For this review, take the finished solid that the model builds, in its own axes (mm). A direction names the side the tool comes from. Give positions to 0.01 mm unless a question says otherwise; leave off trailing zeros. Answer in a Markdown table with one row per item.
```python
from build123d import *

# Parameters (mm, degrees)
SKETCH_1_R          = 23.515666667
SKETCH_1_R_2        = 15.01
EXTRUDE_1_DEPTH     = 3
SKETCH_2_R          = 23.515666667
SKETCH_2_R_2        = 22.515666667
CUT_EXTRUDE_3_DEPTH = 1
FILLET_1_R          = 1
FILLET_2_R          = 1
FILLET_3_R          = 1
CUT_EXTRUDE_4_DEPTH = 34.391213778
SKETCH_5_R          = 21.515666667
SKETCH_5_R_2        = 20.515666667
EXTRUDE_2_DEPTH     = 5
EXTRUDE_3_DEPTH     = 2


with BuildPart() as part:
    # 草图1 → 凸台-拉伸1 (new body)
    with BuildSketch(Plane.XY):
        Circle(SKETCH_1_R)
        Circle(SKETCH_1_R_2, mode=Mode.SUBTRACT)
    extrude(amount=EXTRUDE_1_DEPTH)

    # 草图2 → 切除-拉伸3 (cut)
    with BuildSketch(Plane(origin=(0, 0, 0), x_dir=(-1, 0, 0), z_dir=(0, 0, -1))):
        Circle(SKETCH_2_R)
        Circle(SKETCH_2_R_2, mode=Mode.SUBTRACT)
    extrude(amount=-CUT_EXTRUDE_3_DEPTH, mode=Mode.SUBTRACT)

    # 圆角1
    fillet_1_edges = [part.edges().sort_by_distance(p)[0] for p in [
        (-23.515666667, 0, 3),
    ]]
    fillet(fillet_1_edges, radius=FILLET_1_R)

    # 圆角2
    fillet_2_edges = [part.edges().sort_by_distance(p)[0] for p in [
        (-15.01, 0, 3),
    ]]
    fillet(fillet_2_edges, radius=FILLET_2_R)

    # 圆角3
    fillet_3_edges = [part.edges().sort_by_distance(p)[0] for p in [
        (-15.01, 0, 0),
    ]]
    fillet(fillet_3_edges, radius=FILLET_3_R)

    # 草图3 → 切除-拉伸4 (cut, through all)
    with BuildSketch(Plane.XY.offset(3)):
        with BuildLine():
            Line((1.1, 19.35), (1.1, 17.85))
            ThreePointArc((1.1, 17.85), (0, 16.75), (-1.1, 17.85))
            Line((-1.1, 17.85), (-1.1, 19.35))
            ThreePointArc((-1.1, 19.35), (0, 20.45), (1.1, 19.35))
        make_face()
        with BuildLine():
            Line((7.025641009, 18.063024896), (6.562115518, 16.636440122))
            ThreePointArc((6.562115518, 16.636440122), (5.176034656, 15.930196648), (4.469791182, 17.31627751))
            Line((4.469791182, 17.31627751), (4.933316673, 18.742862284))
            ThreePointArc((4.933316673, 18.742862284), (6.319397535, 19.449105758), (7.025641009, 18.063024896))
        make_face()
        with BuildLine():
            Line((12.263563326, 15.007915064), (11.381885447, 13.794389572))
            ThreePointArc((11.381885447, 13.794389572), (9.845402976, 13.551034656), (9.60204806, 15.087517127))
            Line((9.60204806, 15.087517127), (10.483725938, 16.301042619))
            ThreePointArc((10.483725938, 16.301042619), (12.020208409, 16.544397535), (12.263563326, 15.007915064))
        make_face()
        with BuildLine():
            Line((16.301042619, 10.483725938), (15.087517127, 9.60204806))
            ThreePointArc((15.087517127, 9.60204806), (13.551034656, 9.845402976), (13.794389572, 11.381885447))
            Line((13.794389572, 11.381885447), (15.007915064, 12.263563326))
            ThreePointArc((15.007915064, 12.263563326), (16.544397535, 12.020208409), (16.301042619, 10.483725938))
        make_face()
        with BuildLine():
            Line((18.742862284, 4.933316673), (17.31627751, 4.469791182))
            ThreePointArc((17.31627751, 4.469791182), (15.930196648, 5.176034656), (16.636440122, 6.562115518))
            Line((16.636440122, 6.562115518), (18.063024896, 7.025641009))
            ThreePointArc((18.063024896, 7.025641009), (19.449105758, 6.319397535), (18.742862284, 4.933316673))
        make_face()
        with BuildLine():
            Line((19.35, -1.1), (17.85, -1.1))
            ThreePointArc((17.85, -1.1), (16.75, 0), (17.85, 1.1))
            Line((17.85, 1.1), (19.35, 1.1))
            ThreePointArc((19.35, 1.1), (20.45, 0), (19.35, -1.1))
        make_face()
        with BuildLine():
            Line((18.063024896, -7.025641009), (16.636440122, -6.562115518))
            ThreePointArc((16.636440122, -6.562115518), (15.930196648, -5.176034656), (17.31627751, -4.469791182))
            Line((17.31627751, -4.469791182), (18.742862284, -4.933316673))
            ThreePointArc((18.742862284, -4.933316673), (19.449105758, -6.319397535), (18.063024896, -7.025641009))
        make_face()
        with BuildLine():
            Line((15.007915064, -12.263563326), (13.794389572, -11.381885447))
            ThreePointArc((13.794389572, -11.381885447), (13.551034656, -9.845402976), (15.087517127, -9.60204806))
            Line((15.087517127, -9.60204806), (16.301042619, -10.483725938))
            ThreePointArc((16.301042619, -10.483725938), (16.544397535, -12.020208409), (15.007915064, -12.263563326))
        make_face()
        with BuildLine():
            Line((10.483725938, -16.301042619), (9.60204806, -15.087517127))
            ThreePointArc((9.60204806, -15.087517127), (9.845402976, -13.551034656), (11.381885447, -13.794389572))
            Line((11.381885447, -13.794389572), (12.263563326, -15.007915064))
            ThreePointArc((12.263563326, -15.007915064), (12.020208409, -16.544397535), (10.483725938, -16.301042619))
        make_face()
        with BuildLine():
            Line((4.933316673, -18.742862284), (4.469791182, -17.31627751))
            ThreePointArc((4.469791182, -17.31627751), (5.176034656, -15.930196648), (6.562115518, -16.636440122))
            Line((6.562115518, -16.636440122), (7.025641009, -18.063024896))
            ThreePointArc((7.025641009, -18.063024896), (6.319397535, -19.449105758), (4.933316673, -18.742862284))
        make_face()
        with BuildLine():
            Line((-1.1, -19.35), (-1.1, -17.85))
            ThreePointArc((-1.1, -17.85), (0, -16.75), (1.1, -17.85))
            Line((1.1, -17.85), (1.1, -19.35))
            ThreePointArc((1.1, -19.35), (0, -20.45), (-1.1, -19.35))
        make_face()
        with BuildLine():
            Line((-7.025641009, -18.063024896), (-6.562115518, -16.636440122))
            ThreePointArc((-6.562115518, -16.636440122), (-5.176034656, -15.930196648), (-4.469791182, -17.31627751))
            Line((-4.469791182, -17.31627751), (-4.933316673, -18.742862284))
            ThreePointArc((-4.933316673, -18.742862284), (-6.319397535, -19.449105758), (-7.025641009, -18.063024896))
        make_face()
        with BuildLine():
            Line((-12.263563326, -15.007915064), (-11.381885447, -13.794389572))
            ThreePointArc((-11.381885447, -13.794389572), (-9.845402976, -13.551034656), (-9.60204806, -15.087517127))
            Line((-9.60204806, -15.087517127), (-10.483725938, -16.301042619))
            ThreePointArc((-10.483725938, -16.301042619), (-12.020208409, -16.544397535), (-12.263563326, -15.007915064))
        make_face()
        with BuildLine():
            Line((-16.301042619, -10.483725938), (-15.087517127, -9.60204806))
            ThreePointArc((-15.087517127, -9.60204806), (-13.551034656, -9.845402976), (-13.794389572, -11.381885447))
            Line((-13.794389572, -11.381885447), (-15.007915064, -12.263563326))
            ThreePointArc((-15.007915064, -12.263563326), (-16.544397535, -12.020208409), (-16.301042619, -10.483725938))
        make_face()
        with BuildLine():
            Line((-18.742862284, -4.933316673), (-17.31627751, -4.469791182))
            ThreePointArc((-17.31627751, -4.469791182), (-15.930196648, -5.176034656), (-16.636440122, -6.562115518))
            Line((-16.636440122, -6.562115518), (-18.063024896, -7.025641009))
            ThreePointArc((-18.063024896, -7.025641009), (-19.449105758, -6.319397535), (-18.742862284, -4.933316673))
        make_face()
        with BuildLine():
            Line((-19.35, 1.1), (-17.85, 1.1))
            ThreePointArc((-17.85, 1.1), (-16.75, 0), (-17.85, -1.1))
            Line((-17.85, -1.1), (-19.35, -1.1))
            ThreePointArc((-19.35, -1.1), (-20.45, 0), (-19.35, 1.1))
        make_face()
        with BuildLine():
            Line((-18.063024896, 7.025641009), (-16.636440122, 6.562115518))
            ThreePointArc((-16.636440122, 6.562115518), (-15.930196648, 5.176034656), (-17.31627751, 4.469791182))
            Line((-17.31627751, 4.469791182), (-18.742862284, 4.933316673))
            ThreePointArc((-18.742862284, 4.933316673), (-19.449105758, 6.319397535), (-18.063024896, 7.025641009))
        make_face()
        with BuildLine():
            Line((-15.007915064, 12.263563326), (-13.794389572, 11.381885447))
            ThreePointArc((-13.794389572, 11.381885447), (-13.551034656, 9.845402976), (-15.087517127, 9.60204806))
            Line((-15.087517127, 9.60204806), (-16.301042619, 10.483725938))
            ThreePointArc((-16.301042619, 10.483725938), (-16.544397535, 12.020208409), (-15.007915064, 12.263563326))
        make_face()
        with BuildLine():
            Line((-10.483725938, 16.301042619), (-9.60204806, 15.087517127))
            ThreePointArc((-9.60204806, 15.087517127), (-9.845402976, 13.551034656), (-11.381885447, 13.794389572))
            Line((-11.381885447, 13.794389572), (-12.263563326, 15.007915064))
            ThreePointArc((-12.263563326, 15.007915064), (-12.020208409, 16.544397535), (-10.483725938, 16.301042619))
        make_face()
        with BuildLine():
            Line((-4.933316673, 18.742862284), (-4.469791182, 17.31627751))
            ThreePointArc((-4.469791182, 17.31627751), (-5.176034656, 15.930196648), (-6.562115518, 16.636440122))
            Line((-6.562115518, 16.636440122), (-7.025641009, 18.063024896))
            ThreePointArc((-7.025641009, 18.063024896), (-6.319397535, 19.449105758), (-4.933316673, 18.742862284))
        make_face()
    extrude(amount=-CUT_EXTRUDE_4_DEPTH, mode=Mode.SUBTRACT)

    # 草图5 → 凸台-拉伸2 (add)
    with BuildSketch(Plane(origin=(0, 0, 0), x_dir=(-1, 0, 0), z_dir=(0, 0, -1))):
        with Locations(Location((0, 0, 0), (0, 0, 180))):
            Circle(SKETCH_5_R)
        Circle(SKETCH_5_R_2, mode=Mode.SUBTRACT)
    extrude(amount=EXTRUDE_2_DEPTH)

    # 草图6 → 凸台-拉伸3 (add)
    with BuildSketch(Plane(origin=(0, 0, -5), x_dir=(-1, 0, 0), z_dir=(0, 0, -1))):
        with BuildLine():
            Line((-16.26911987, -9.852722397), (-18.353991972, -11.115339319))
            ThreePointArc((-18.353991972, -11.115339319), (-20.274508623, -7.025958268), (-21.29621173, -2.625101039))
            Line((-21.29621173, -2.625101039), (-18.877126128, -2.326909783))
            ThreePointArc((-18.877126128, -2.326909783), (-17.971480624, -6.227863532), (-16.26911987, -9.852722397))
        make_face()
        with BuildLine():
            Line((-9.852722397, 16.26911987), (-11.115339319, 18.353991972))
            ThreePointArc((-11.115339319, 18.353991972), (-7.025958268, 20.274508623), (-2.625101039, 21.29621173))
            Line((-2.625101039, 21.29621173), (-2.326909783, 18.877126128))
            ThreePointArc((-2.326909783, 18.877126128), (-6.227863532, 17.971480624), (-9.852722397, 16.26911987))
        make_face()
        with BuildLine():
            Line((16.26911987, 9.852722397), (18.353991972, 11.115339319))
            ThreePointArc((18.353991972, 11.115339319), (20.274508623, 7.025958268), (21.29621173, 2.625101039))
            Line((21.29621173, 2.625101039), (18.877126128, 2.326909783))
            ThreePointArc((18.877126128, 2.326909783), (17.971480624, 6.227863532), (16.26911987, 9.852722397))
        make_face()
        with BuildLine():
            Line((9.852722397, -16.26911987), (11.115339319, -18.353991972))
            ThreePointArc((11.115339319, -18.353991972), (7.025958268, -20.274508623), (2.625101039, -21.29621173))
            Line((2.625101039, -21.29621173), (2.326909783, -18.877126128))
            ThreePointArc((2.326909783, -18.877126128), (6.227863532, -17.971480624), (9.852722397, -16.26911987))
        make_face()
    extrude(amount=-EXTRUDE_3_DEPTH)


solid = part.part
```
1. Mouldability with a two-part tool opening along X and no side actions: class faces 1 (the face through (0, -23, 1)), 2 (the face through (15.703, 10.049, 1.521)), 3 (the face through (-6, -19, -3)) as released by +X, released by -X, zero draft, split by the parting line, or undercut.
Values:
| item | result |
|---|---|
| face 1 | zero draft |
| face 2 | undercut |
| face 3 | undercut |
2. For faces 4 (the face through (10.049, -15.703, 1.521)), 5 (the face through (-6.17, -17.99, -4.01)), 6 (the face through (-19, 6, -3)), list the 3-axis set-ups (+Z, -Z, +X, -X, +Y, -Y) from which the entire face can be reached by the end or side of a thin tool; tool diameter is ignored.
Values:
| item | result |
|---|---|
| face 4 | +Z, -Z |
| face 5 | -Z |
| face 6 | none |
3. We need section A-A, the plane x = 0. Count the separate pieces of the cut face and the enclosed holes in it, and give its area (3 significant figures).
Values:
| item | result |
|---|---|
| separate pieces | 4 |
| enclosed holes | 0 |
| area | 35.5 mm^2 |
4. Wall thickness on line 1 (Y direction, x = 0, z = 1.8); line 2 (X direction, y = 1, z = 1.25); line 3 (Y direction, x = 0, z = -1.8): over which ranges is each line inside the solid? List them lowest first. Write a range as [from, to].
Values:
| item | result |
|---|---|
| line 1 | y = [-23.52, -20.45], [-16.75, -15.01], [15.01, 16.75], [20.45, 23.52] |
| line 2 | x = [-23.49, -19.81], [-17.39, -14.98], [14.98, 17.39], [19.81, 23.49] |
| line 3 | y = [-21.52, -20.52], [20.52, 21.52] |
5. Clearance check with flat-ended pins moving along their axes: pin 1 (1 mm diameter, centred on x = -13, y = 13, fed in from -Z); pin 2 (1.6 mm diameter, centred on y = 18.5, z = 1.5, fed in from +X); pin 3 (0.8 mm diameter, centred on x = -18.5, z = 1, fed in from -Y). State where each tip first meets the part, or that it passes through.
Values:
| item | result |
|---|---|
| pin 1 | stops at z = 0 |
| pin 2 | stops at x = 15.48 |
| pin 3 | stops at y = -15.01 |
